The listing builds one solid part. Answer for the finished solid, in the listing's coordinates (mm). A direction names the side the tool comes from. Give positions to 0.01 mm unless a question says otherwise; leave off trailing zeros. Order: outer loops, then holes, each group sorted by start corner. A loop starts at its lowest first (then second) coordinate and runs counter-clockwise, first axis right, second up. Notation, with made-up numbers: (31, 84.5) - (36, 84.5) arc R20 ccw to (36, 109.5) - close; hole circle Ø9 at (59, 42). An arc over 180 degrees is marked (long way). Answer in a Markdown table with one row per item.
from build123d import *

# Parameters (mm, degrees)
F0_W           = 101.6
F0_H           = 38.1
F0_R           = 6.35
F1_DEPTH       = 12.7
F3_DEPTH       = 12.7
F4_D           = 11.90625
F4_CBORE_D     = 25.4
F4_CBORE_DEPTH = 6.35
F5_W           = 38.1
F5_H           = 3.175
F6_DEPTH       = 38.101
F9_R           = 3.175
F9_R_2         = 3.17499


# Not quite as in the source:
# - a fillet or chamfer is up to 0.001 mm smaller than in the source, because OpenCascade refuses the exact size
# - a feature of the source that left no trace in its solid (it failed there, or was rolled back) is left out
# - a length typed as a fraction of an inch, garbled in the dataset ("3 / 203.2 mm" for 3/8 in), is restored


with BuildPart() as f1:
    # F0 (on Top) → F1 (new body)
    with BuildSketch(Plane.XY):
        with Locations((12.3613710271, 3.3725141548)):
            Rectangle(F0_W, F0_H)
        with Locations((-25.7386289729, 9.7225141548)):
            Circle(F0_R, mode=Mode.SUBTRACT)
        with Locations((50.4613710271, 9.7225141548)):
            Circle(F0_R, mode=Mode.SUBTRACT)
    extrude(amount=F1_DEPTH)

    # F2 (on face) → F3 (join)
    with BuildSketch(Plane.XZ.offset(15.6774858452)):
        with BuildLine():
            Line((-6.6886289729, 38.1), (-6.6886289729, 12.7))
            Line((-6.6886289729, 12.7), (31.4113710271, 12.7))
            Line((31.4113710271, 12.7), (31.4113710271, 38.1))
            ThreePointArc((31.4113710271, 38.1), (12.3613710271, 57.15), (-6.6886289729, 38.1))
        make_face()
    extrude(amount=-F3_DEPTH)

    # F4 (through all)
    with Locations(Plane.XZ.offset(15.6774858452)):
        with Locations((12.3613710271, 38.1)):
            CounterBoreHole(F4_D / 2, F4_CBORE_D / 2, F4_CBORE_DEPTH)

    # F5 (on face) → F6 (cut, through all)
    with BuildSketch(Plane(origin=(0, 22.4225141548, 0), x_dir=(-1, 0, 0), z_dir=(0, 1, 0))):
        with Locations((-12.3613710271, 1.5875)):
            Rectangle(F5_W, F5_H)
    extrude(amount=-F6_DEPTH, mode=Mode.SUBTRACT)

    # F8: union 

    # F9 (call 1 of 3: OpenCascade refuses the feature's edges together)
    f9_edges = [f1.edges().sort_by_distance(p)[0] for p in [
        (63.161371, -15.677486, 6.35),
        (63.161371, 22.422514, 6.35),
        (-38.438629, -15.677486, 6.35),
        (-38.438629, 22.422514, 6.35),
        (12.361371, 22.422514, 12.7),
        (63.161371, 3.372514, 12.7),
        (-38.438629, 3.372514, 12.7),
        (47.286371, -15.677486, 12.7),
        (-22.563629, -15.677486, 12.7),
        (12.361371, -2.977486, 12.7),
        (31.411371, -9.327486, 12.7),
        (-6.688629, -9.327486, 12.7),
        (31.411371, -15.677486, 25.4),
        (12.361371, -15.677486, 57.15),
        (-6.688629, -15.677486, 25.4),
    ]]
    fillet(f9_edges, radius=F9_R)

    # F9#2 (call 2 of 3) (radius 3.175 in the source; OpenCascade refuses exactly that, so slightly less here)
    f9_2_edges = [f1.edges().sort_by_distance(p)[0] for p in [
        (-6.688629, 3.372514, 3.175),
    ]]
    fillet(f9_2_edges, radius=F9_R_2)

    # F9#3 (call 3 of 3) (radius 3.175 in the source; OpenCascade refuses exactly that, so slightly less here)
    f9_3_edges = [f1.edges().sort_by_distance(p)[0] for p in [
        (31.411371, 3.372514, 3.175),
    ]]
    fillet(f9_3_edges, radius=F9_R_2)


solid = f1.part
Item 1: Which of the six approach directions +Z, -Z, +X, -X, +Y, -Y give full straight-line access (tool end or side, diameter ignored) to faces 1 (the face through (-5.783, 3.106, 2.22)), 2 (the face through (-5.734, -14.772, 26.832)), 3 (the face through (47.46, -14.77, 11.75)), 4 (the face through (16, -2.977, 32)), 5 (the face through (-6.689, -8, 27))?
Answer block:
| item | result |
|---|---|
| face 1 | -Z, +Y, -Y |
| face 2 | +Z, -X, -Y |
| face 3 | +Z, +X, -Y |
| face 4 | +Z, +X, -X, +Y |
| face 5 | +Z, -X, +Y, -Y |
Item 2: Find section D-D on x = 41. Write down the section's boundary in (y, z) (3 decimals).
Answer block:
| item | result |
|---|---|
| outline | (-15.677, 0) - (22.423, 0) - (22.423, 9.525) arc R3.175 ccw to (19.248, 12.7) - (-12.502, 12.7) arc R3.175 ccw to (-15.677, 9.525) - close |
Item 3: Determine the mould class of faces 6 (the face through (62.207, 21.517, 4.829)), 7 (the face through (19.2, -12.5, 48.8)), 8 (the face through (-37.5, 21.5, 4.8)) for opening direction X: pulls with the +X half, pulls with the -X half, needs draft (parallel to the pull), parting line crosses it, or undercut.
Answer block:
| item | result |
|---|---|
| face 6 | pulls with the +X half |
| face 7 | undercut |
| face 8 | pulls with the -X half |
Item 4: Each of these flat-tipped pins is pushed along its axis until it touches: P1, Ø7.5, axis at y = -5.5, z = 31.5, coming from the -X side; P2, Ø5, axis at y = -7.5, z = 31.5, coming from the +X side; P3, Ø12.5, axis at x = 18, z = 37, coming from the -Y side. Where does it stop, or does it pass through?
Answer block:
| item | result |
|---|---|
| P1 | x = -6.69 |
| P2 | x = 31.41 |
| P3 | y = -9.33 |
Item 5: Find section C-C on z = 28.5. Write down the section's boundary in (x, y) (3 decimals).
Answer block:
| item | result |
|---|---|
| outline | (-6.689, -12.502) arc R3.175 ccw to (-3.514, -15.677) - (4.047, -15.677) - (4.047, -9.327) - (20.676, -9.327) - (20.676, -15.677) - (28.236, -15.677) arc R3.175 ccw to (31.411, -12.502) - (31.411, -2.977) - (-6.689, -2.977) - close |
Item 6: Find section B-B on x = -26. Write down the section's boundary in (y, z) (3 decimals).
Answer block:
| item | result |
|---|---|
| outline | (-15.677, 0) - (3.378, 0) - (3.378, 12.7) - (-12.502, 12.7) arc R3.175 ccw to (-15.677, 9.525) - close; (16.067, 0) - (22.423, 0) - (22.423, 9.525) arc R3.175 ccw to (19.248, 12.7) - (16.067, 12.7) - close |
Item 7: Consider line 1 (X direction, y = 11, z = 10); line 2 (Z direction, x = 57.5, y = 18); line 3 (Y direction, x = 2, z = 37.5). Determine where each line is inside the solid, lowest interval first.
Answer block:
| item | result |
|---|---|
| line 1 | -38.4 to -31.96, -19.52 to 44.24, 56.68 to 63.13 |
| line 2 | 0 to 12.7 |
| line 3 | -9.33 to -2.98 |
